Autodesk Inventor part; units mm, degrees
ref_plane "YZ Plane" through (0, 0, 0) normal (1, 0, 0) x (0, 1, 0)
ref_plane "XZ Plane" through (0, 0, 0) normal (0, 1, 0) x (-1, 0, 0)
ref_plane "XY Plane" through (0, 0, 0) normal (0, 0, 1) x (1, 0, 0)
sketch "スケッチ1" plane through (0, 0, 0) normal (0, 1, 0) x (-1, 0, 0)
  circle A0 centre (0, 0) radius 4
  dimension "d0" = 8
extrude "押し出し1" add sketch "スケッチ1" along normal blind 91
sketch "スケッチ2" plane through (0, 0, 0) normal (0, -1, 0) x (1, 0, 0)
  point P0 (0, 0)
sketch "スケッチ3" plane through (0, 91, 0) normal (0, 1, 0) x (1, 0, 0)
  point P0 (0, 0)
hole "穴1" at (0, 91, 0) direction (0, -1, 0) diameter 3.242 depth 30 tip angle 118 countersink diameter 4 countersink angle 90
hole "穴2" at (0, 0, 0) direction (0, 1, 0) diameter 3.242 depth 30 tip angle 118 countersink diameter 4 countersink angle 90
properties part number "p8ALshaft" material "アルミニウム 2014-T4"
Design review of the part built by this model. Coordinates are the model's own, in mm. A direction names the side the tool comes from. Coordinates: 2 decimals unless noted, no trailing zeros. Loops run counter-clockwise (first coordinate to the right, second up) from the corner with the lowest first, then second, coordinate; pieces in that order, holes last.
Item 1: Add section B-B (y = 34). Write out the cut boundary in (x, z).
Completed:
outline: circle Ø8 at (0, 0)
Item 2: Add section C-C (z = -3). Write out the cut boundary in (x, y), and give its area (3 significant figures).
Completed:
outline: (-2.65, 0) - (2.65, 0) - (2.65, 91) - (-2.65, 91) - close
area: 482 mm2
Item 3: Draft analysis for pull direction X (two halves, no side actions). For faces 1 (the cylindrical face through (1.438, 15.397, -0.748)), 2 (the cylindrical face through (0.867, 44.863, 3.905)), 3 (the flat face through (2, 0, -1)), state which applies: pulls with the +X half, pulls with the -X half, needs draft (parallel to the pull), parting line crosses it, or undercut.
Completed:
face 1: undercut
face 2: parting line crosses it
face 3: needs draft
Item 4: For faces 4 (the flat face through (2, 91, -1)), 5 (the cylindrical face through (1.438, 75.603, 0.748)), list the 3-axis set-ups (+Z, -Z, +X, -X, +Y, -Y) from which the entire face can be reached by the end or side of a thin tool; tool diameter is ignored.
Completed:
face 4: +Z, -Z, +X, -X, +Y
face 5: +Y
Item 5: Clearance check with flat-ended pins moving along their axes: pin 1 (2.5 mm diameter, centred on x = 0, z = 0, fed in from -Y); pin 2 (2 mm diameter, centred on y = 38, z = -2.5, fed in from +X); pin 3 (2 mm diameter, centred on y = 56.5, z = 2, fed in from -X). State where each tip first meets the part, or that it passes through.
Completed:
pin 1: stops at y = 30.22
pin 2: stops at x = 3.71
pin 3: stops at x = -3.87
Item 6: Wall thickness on L1, parallel to Z at x = 0, y = 19.25; L2, parallel to X at y = 21.5, z = 0.25; L3, parallel to X at y = 61.5, z = -1.25: over which ranges is each line inside the solid? List them lowest first.
Completed:
L1: z = -4 to -1.62, 1.62 to 4
L2: x = -3.99 to -1.6, 1.6 to 3.99
L3: x = -3.8 to -1.03, 1.03 to 3.8
Item 7: Add section A-A (y = 68). Write out the cut boundary in (x, z), and give its area (3 significant figures).
Completed:
outline: circle Ø8 at (0, 0); hole circle Ø3.24 at (0, 0)
area: 42.0 mm2
Item 8: Add section D-D (x = 2.75). Write out the cut boundary in (y, z).
Completed:
outline: (0, -2.9) - (91, -2.9) - (91, 2.9) - (0, 2.9) - close
